Study the drawing (mm; zero at the part's minimum x, y, z) and answer. A direction names the side the tool comes from. Coordinates: 2 decimals unless noted, no trailing zeros. Loops run counter-clockwise (first coordinate to the right, second up) from the corner with the lowest first, then second, coordinate; pieces in that order, holes last. Notation, with made-up numbers: (31.25, 59) -> (86.25, 59) arc R27 ccw to (86.25, 88) -> close; hole circle Ø1 at (-22, 13). An arc over 180 degrees is marked (long way). Answer as a JSON object with one key per item and string values. Group by question number.
Q1. For the marked faces 1 and 2, determine the directions among +Z, -Z, +X, -X, +Y, -Y from which every point of the face is accessible in a straight line to the end or side of a thin tool.
Q2. The part is cut by section B-B on y = 6.5. State how many separate pieces and enclosed holes the cut face has, and give its area (3 significant figures).
Q3. Determine the mould class of the marked faces 3, 4 and 5 for opening direction Z: released by +Z, released by -Z, zero draft, split by the parting line, or undercut.
Q4. The part is cut by section A-A on x = 52.5. Write down the section's boundary in (y, z), and give its area (3 significant figures).
Q5. The part is cut by section C-C on z = 30. Write down the section's boundary in (x, y).
Q6. Straight lines are drawn through the part: line 1 along X through (y, z) = (8, 43) (1 decimal); line 2 along Z through (x, y) = (44, 9.5); line 3 along X through (y, z) = (1.75, 20). For each, find the intervals that lie inside material, in ascending order. Write a range as [from, to].
Q7. Each of these flat-tipped pins is pushed along its axis until it touches: P1, Ø1.5, axis at y = 6, z = 50, coming from the +X side; P2, Ø6, axis at x = 56.5, y = 2.5, coming from the -Z side; P3, Ø2, axis at x = 70, y = 2.5, coming from the +Z side. Where does it stop, or does it pass through?
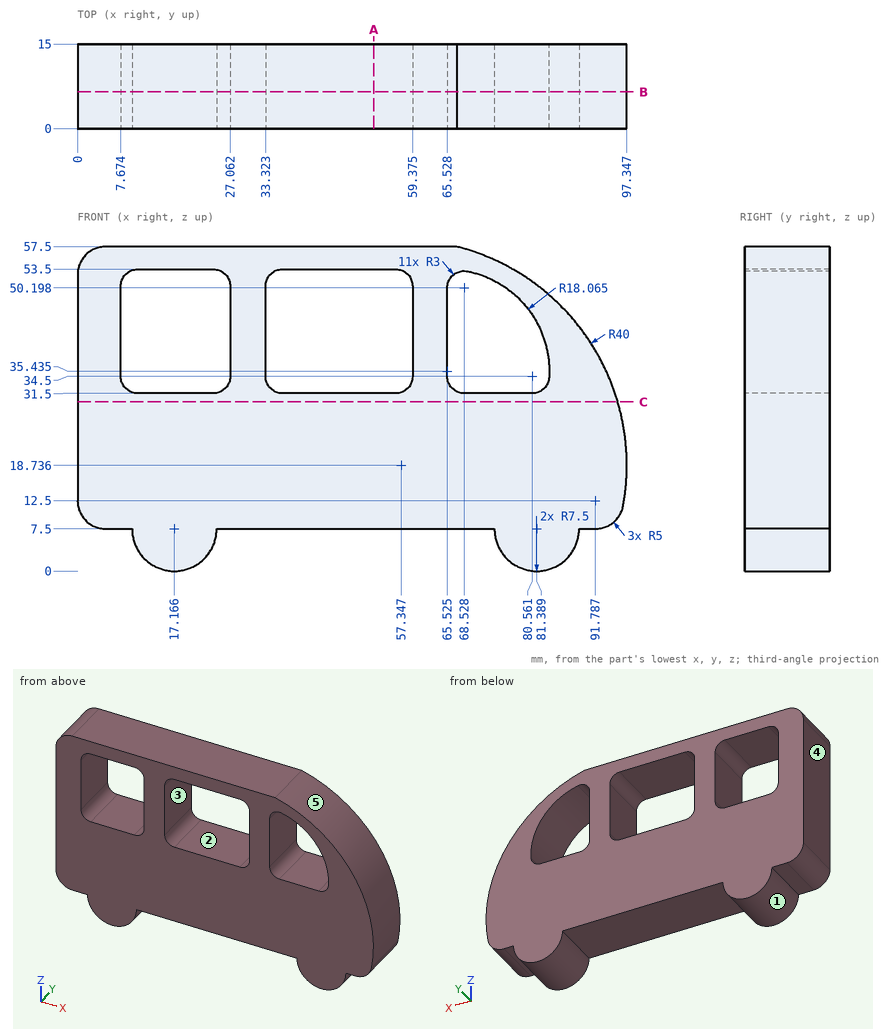
Final values:
{
 "1": {"face 1": "-Z, +Y, -Y", "face 2": "+Y, -Y"},
 "2": {"separate pieces": "1", "enclosed holes": "3", "area": "3,420 mm2"},
 "3": {"face 3": "undercut", "face 4": "zero draft", "face 5": "split by the parting line"},
 "4": {"outline": "(0, 7.5) -> (15, 7.5) -> (15, 31.5) -> (0, 31.5) -> close; (0, 53.5) -> (15, 53.5) -> (15, 57.5) -> (0, 57.5) -> close", "area": "420 mm2"},
 "5": {"outline": "(0, 0) -> (95.73, 0) -> (95.73, 15) -> (0, 15) -> close"},
 "6": {"line 1": "x = [0, 7.7], [27.1, 33.3], [59.4, 65.5], [81.9, 89.1]", "line 2": "z = [7.5, 31.5], [53.5, 57.5]", "line 3": "x = [0, 97.33]"},
 "7": {"P1": "stops at x = 83.21", "P2": "stops at z = 7.5", "P3": "stops at z = 57"}
}
